from build123d import *

# Parameters (mm, degrees)
BASEHEAD_DEPTH = 20
COLLAR_START   = -5.15
COLLARSKE_R    = 14
COLLAR_DEPTH   = 5.15
HEADFILLET_R   = 0.8


# Read off the part's stored shape, not the designer's step: HeadChamfer
with BuildPart() as part:
    # SquareSke → BaseHead (new body)
    with BuildSketch(Plane(origin=(0, 0, 0), x_dir=(0, 0, -1), z_dir=(1, 0, 0))):
        with BuildLine():
            Line((13.90189895, -1.654450236), (1.654450236, -13.90189895))
            ThreePointArc((1.654450236, -13.90189895), (0, -14), (-1.654450236, -13.90189895))
            Line((-1.654450236, -13.90189895), (-13.90189895, -1.654450236))
            ThreePointArc((-13.90189895, -1.654450236), (-14, 0), (-13.90189895, 1.654450236))
            Line((-13.90189895, 1.654450236), (-1.654450236, 13.90189895))
            ThreePointArc((-1.654450236, 13.90189895), (0, 14), (1.654450236, 13.90189895))
            Line((1.654450236, 13.90189895), (13.90189895, 1.654450236))
            ThreePointArc((13.90189895, 1.654450236), (14, 0), (13.90189895, -1.654450236))
        make_face()
    extrude(amount=BASEHEAD_DEPTH)

    # HeadChamfer outline → HeadChamfer (revolve, cut)
    with BuildSketch(Plane.YX):
        Polygon((14.000000007, 1.732050812), (11, 0), (14.000000007, 0), align=None)
    revolve(axis=Axis((0, 0, 0), (1, 0, 0)), mode=Mode.SUBTRACT)

    # HeadChamfer 2 outline → HeadChamfer 2 (revolve)
    with BuildSketch(Plane.YX):
        with BuildLine():
            Line((5.221450167, 89.7), (5.221450173, 92.999999995))
            ThreePointArc((5.221450173, 92.999999995), (2.79569052, 94.482893893), (0, 95))
            Line((0, 95), (0, 20))
            Line((0, 20), (8.520797289, 20))
            Line((8.520797289, 20), (8.520797289, 86.400652878))
            Line((8.520797289, 86.400652878), (5.221450167, 89.7))
        make_face()
    revolve(axis=Axis((0, 0, 0), (1, 0, 0)))

    # CollarSke → Collar (add)
    with BuildSketch(Plane(origin=(20, 0, 0), x_dir=(0, 0, -1), z_dir=(1, 0, 0)).offset(COLLAR_START)):
        with Locations(Location((0, 0, 0), (0, 0, 173.213210702))):
            Circle(COLLARSKE_R)
    extrude(amount=COLLAR_DEPTH)

    # HeadFillet
    headfillet_edges = [part.edges().sort_by_distance(p)[0] for p in [
        (20, -8.520797289, 0),
    ]]
    fillet(headfillet_edges, radius=HEADFILLET_R)


solid = part.part
The model under review builds one solid part; all positions refer to its coordinate system, in mm. A direction names the side the tool comes from. Round coordinates to 2 decimals unless told otherwise and drop trailing zeros. Loops run counter-clockwise (first coordinate to the right, second up) from the corner with the lowest first, then second, coordinate; pieces in that order, holes last. Notation, with made-up numbers: (8.5, 40) -> (18.5, 40) arc R31 ccw to (18.5, 73) -> close; hole circle Ø4 at (-23, -35). An arc over 180 degrees is marked (long way). One line per question, with ' | ' between items. Start each with the question number.
Item 1: Machinability: for faces 1 (the face through (7.321, -7.864, 7.692)), 2 (the face through (54.06, 8.127, 2.559)), 3 (the face through (7.321, -7.692, -7.864)), 4 (the face through (14.85, 9, -9)), which of the approach directions +Z, -Z, +X, -X, +Y, -Y give a long, thin tool a straight path to every point of the face, cutting with its end or side? Answer none if there is none.
Item 2: Add section D-D, the plane x = 68. Write out the cut boundary in (y, z), then the cut area to 3 significant figures.
Item 3: Wall thickness on line 1 along X through (y, z) = (10, -2); line 2 along Z through (x, y) = (51, 0); line 3 along X through (y, z) = (-9.75, -6): over which ranges is each line inside the solid? List them lowest first. Write a range as [from, to].
Item 4: Add section A-A, the plane z = 0. Write out the cut boundary in (x, y).
Item 5: For pin 1 (10 mm diameter, centred on y = 1.5, z = -6.5, fed in from +X); pin 2 (2 mm diameter, centred on y = -10, z = -2.5, fed in from +X); pin 3 (10 mm diameter, centred on y = 8.5, z = 5, fed in from +X), all flat-tipped, find the tip position at first contact; note any pin that passes through.
Item 6: Add section B-B, the plane x = 13. Write out the cut boundary in (y, z).
Return value:
1) face 1: +Z, -X, -Y | face 2: +X | face 3: -Z, -X, -Y | face 4: -Z, -X, +Y
2) outline: circle Ø17.04 at (0, 0) | area: 228 mm2
3) line 1: x = [0, 20] | line 2: z = [-8.52, 8.52] | line 3: x = [14.85, 20]
4) outline: (0, -11) -> (1.73, -14) -> (20, -14) -> (20, -9.32) arc R0.8 cw to (20.8, -8.52) -> (86.4, -8.52) -> (89.7, -5.22) -> (93, -5.22) arc R7.82 ccw to (93, 5.22) -> (89.7, 5.22) -> (86.4, 8.52) -> (20.8, 8.52) arc R0.8 cw to (20, 9.32) -> (20, 14) -> (1.73, 14) -> (0, 11) -> close
5) pin 1: stops at x = 94.82 | pin 2: stops at x = 20 | pin 3: stops at x = 93.3
6) outline: (-13.9, -1.65) -> (-1.65, -13.9) arc R14 ccw to (1.65, -13.9) -> (13.9, -1.65) arc R14 ccw to (13.9, 1.65) -> (1.65, 13.9) arc R14 ccw to (-1.65, 13.9) -> (-13.9, 1.65) arc R14 ccw to start
